from build123d import *

# Parameters (mm, degrees)
CYLINDER001_R          = 2.5
CYLINDER001_DEPTH      = 30
CYLINDER001_ROLL_ANGLE = -90
BOX001_W               = 25
BOX001_H               = 4
BOX001_DEPTH           = 10
BOX002_W               = 20
BOX002_H               = 5
BOX002_DEPTH           = 10
BOX003_W               = 20
BOX003_H               = 5
BOX003_DEPTH           = 10
CYLINDER_R             = 10
CYLINDER_DEPTH         = 10
BOX_W                  = 45
BOX_H                  = 30
BOX_DEPTH              = 10


with BuildPart() as cylinder001:
    # Cylinder001 → Cylinder001 (new body)
    with BuildSketch(Plane.XY):
        Circle(CYLINDER001_R)
    extrude(amount=CYLINDER001_DEPTH)


with BuildPart() as cylinder001_1:
    # Cylinder001 roll: moved
    add(cylinder001.part.rotate(Axis((0, 0, 0), (1, 0, 0)), CYLINDER001_ROLL_ANGLE))


with BuildPart() as cylinder001_2:
    # Cylinder001 placement: moved
    add(cylinder001_1.part.moved(Location((-20, -15, 0))))


with BuildPart() as cube001:
    # Box001 → Box001 (new body)
    with BuildSketch(Plane(origin=(-30, -2, -5), x_dir=(1, 0, 0), z_dir=(0, 0, 1))):
        with Locations((12.5, 2)):
            Rectangle(BOX001_W, BOX001_H)
    extrude(amount=BOX001_DEPTH)


with BuildPart() as cube002:
    # Box002 → Box002 (new body)
    with BuildSketch(Plane(origin=(-30, -15, -5), x_dir=(1, 0, 0), z_dir=(0, 0, 1))):
        with Locations((10, 2.5)):
            Rectangle(BOX002_W, BOX002_H)
    extrude(amount=BOX002_DEPTH)


with BuildPart() as cube003:
    # Box003 → Box003 (new body)
    with BuildSketch(Plane(origin=(-30, 10, -5), x_dir=(1, 0, 0), z_dir=(0, 0, 1))):
        with Locations((10, 2.5)):
            Rectangle(BOX003_W, BOX003_H)
    extrude(amount=BOX003_DEPTH)


with BuildPart() as negative_fusion:
    # Cylinder → Cylinder (new body)
    with BuildSketch(Plane.XY.offset(-5)):
        Circle(CYLINDER_R)
    extrude(amount=CYLINDER_DEPTH)

    # Fusion: union Cylinder001, Cube001, Cube002, Cube003
    add(cylinder001_2.part)
    add(cube001.part)
    add(cube002.part)
    add(cube003.part)


with BuildPart() as cut:
    # Box → Box (new body)
    with BuildSketch(Plane(origin=(-30, -15, -5), x_dir=(1, 0, 0), z_dir=(0, 0, 1))):
        with Locations((22.5, 15)):
            Rectangle(BOX_W, BOX_H)
    extrude(amount=BOX_DEPTH)

    # Cut: cut Negative Fusion
    add(negative_fusion.part, mode=Mode.SUBTRACT)


solid = cut.part
Design review of the part built by this model. Coordinates are the model's own, in mm. A direction names the side the tool comes from. Round coordinates to 2 decimals unless told otherwise and drop trailing zeros. Write each loop counter-clockwise with the first axis right and the second up, starting at its lowest first coordinate (ties: lowest second). Pieces come first, ordered by that corner, then holes. Notation, with made-up numbers: (20, 68.5) - (62, 68.5) arc R21 cw to (62, 83.5) - close; hole circle Ø2 at (48, 52.25). An arc over 180 degrees is marked (long way). Use a Markdown table: item, result. Add a question column.
1. We need section D-D (x = 0). State the section outline as (y, z) points, then the cut area to 3 significant figures.
2. We need section A-A (z = 0). State the section outline as (x, y) points, then the cut area to 3 significant figures.
3. For faces 5 (the face through (-22.4, 10, -1.2)), 6 (the face through (-22, -2, -2)), 7 (the face through (-22.4, -10, -1.2)), 8 (the face through (-30, 6, 0)), 9 (the face through (-22.5, -6.1, -0.1)), list the 3-axis set-ups (+Z, -Z, +X, -X, +Y, -Y) from which the entire face can be reached by the end or side of a thin tool; tool diameter is ignored.
4. Mouldability with a two-part tool opening along Z and no side actions: class faces 1 (the face through (-22, 2, -2)), 2 (the face through (-7.8, -6.5, -5)), 3 (the face through (-7.8, -6.5, 5)), 4 (the face through (-22.5, 5.9, -0.1)) as +Z half, -Z half, draft (parallel to the pull), parting line (faces both ways), or undercut.
5. Wall thickness on probe 1 along Y at (x, z) = (0, 0); probe 2 along Y at (x, z) = (-25, -3.5); probe 3 along X at (y, z) = (-3.25, -0.5): over which ranges is each line inside the solid? List them lowest first.
6. We need section B-B (y = 7). State the section outline as (x, z) points.
7. Clearance check with flat-ended pins moving along their axes: pin 1 (2.5 mm diameter, centred on y = -13, z = -2, fed in from -X); pin 2 (4 mm diameter, centred on x = -20, z = 0, fed in from +Y); pin 3 (3 mm diameter, centred on x = -18, z = -1.5, fed in from +Y). State where each tip first meets the part, or that it passes through.
8. We need section C-C (x = -24.5). State the section outline as (y, z) points, then the cut area to 3 significant figures.
Output:
| question | item | result |
|---|---|---|
| 1 | outline | (-15, -5) - (-10, -5) - (-10, 5) - (-15, 5) - close; (10, -5) - (15, -5) - (15, 5) - (10, 5) - close |
| 1 | area | 100 mm2 |
| 2 | outline | (-30, -10) - (-22.5, -10) - (-22.5, -2) - (-30, -2) - close; (-30, 2) - (-22.5, 2) - (-22.5, 10) - (-30, 10) - close; (-17.5, -10) - (-10, -10) - (-10, -15) - (15, -15) - (15, 15) - (-10, 15) - (-10, 10) - (-17.5, 10) - (-17.5, 2) - (-9.8, 2) arc R10 cw (long way) to (-9.8, -2) - (-17.5, -2) - close |
| 2 | area | 676 mm2 |
| 3 | face 5 | +Z, -Z, -X, +Y |
| 3 | face 6 | +Z, -Z, -X |
| 3 | face 7 | +Z, -Z, -X, -Y |
| 3 | face 8 | +Z, -Z, -X, +Y, -Y |
| 3 | face 9 | +Y, -Y |
| 4 | face 1 | draft |
| 4 | face 2 | -Z half |
| 4 | face 3 | +Z half |
| 4 | face 4 | undercut |
| 5 | probe 1 | y = -15 to -10, 10 to 15 |
| 5 | probe 2 | y = -10 to -2, 2 to 10 |
| 5 | probe 3 | x = -30 to -22.45, -17.55 to -9.46, 9.46 to 15 |
| 6 | outline | (-30, -5) - (-7.14, -5) - (-7.14, 5) - (-30, 5) - close; (7.14, -5) - (15, -5) - (15, 5) - (7.14, 5) - close; hole circle Ø5 at (-20, 0) |
| 7 | pin 1 | stops at x = -10 |
| 7 | pin 2 | passes through |
| 7 | pin 3 | stops at y = 10 |
| 8 | outline | (-10, -5) - (-2, -5) - (-2, 5) - (-10, 5) - close; (2, -5) - (10, -5) - (10, 5) - (2, 5) - close |
| 8 | area | 160 mm2 |
